from build123d import *

# Parameters (mm, degrees)
SKETCH1_W          = 300
SKETCH1_H          = 150
BLOCK_DEPTH        = 19.05
SKETCH3_W          = 250
SKETCH3_H          = 25
CUT_EXTRUDE2_DEPTH = 39.961179
SKETCH6_W          = 125
SKETCH6_H          = 20
CUT_EXTRUDE5_DEPTH = 20.05
SKETCH7_W          = 80
SKETCH7_H          = 50
CUT_EXTRUDE6_DEPTH = 20.05
SKETCH8_R          = 2
CUT_EXTRUDE7_DEPTH = 20.05


with BuildPart() as part:
    # Sketch1 → block (new body)
    with BuildSketch(Plane.XY):
        with Locations((150, 75)):
            Rectangle(SKETCH1_W, SKETCH1_H)
    extrude(amount=-BLOCK_DEPTH)

    # Sketch3 → Cut-Extrude2 (cut)
    with BuildSketch(Plane.XY):
        with Locations((150, 117.5)):
            Rectangle(SKETCH3_W, SKETCH3_H)
    extrude(amount=-CUT_EXTRUDE2_DEPTH, mode=Mode.SUBTRACT)

    # Sketch6 → Cut-Extrude5 (cut, through all)
    with BuildSketch(Plane.XY):
        with Locations((212.5, 95)):
            Rectangle(SKETCH6_W, SKETCH6_H)
    extrude(amount=-CUT_EXTRUDE5_DEPTH, mode=Mode.SUBTRACT)

    # Sketch7 → Cut-Extrude6 (cut, through all)
    with BuildSketch(Plane.XY):
        with Locations((200, 25)):
            Rectangle(SKETCH7_W, SKETCH7_H)
    extrude(amount=-CUT_EXTRUDE6_DEPTH, mode=Mode.SUBTRACT)

    # Sketch8 → Cut-Extrude7 (cut, through all)
    with BuildSketch(Plane.XY):
        with Locations((37.5875, 139.35)):
            Circle(SKETCH8_R)
        with Locations((82.0375, 139.35)):
            Circle(SKETCH8_R)
        with Locations((37.5875, 91.95)):
            Circle(SKETCH8_R)
        with Locations((82.0375, 91.95)):
            Circle(SKETCH8_R)
    extrude(amount=-CUT_EXTRUDE7_DEPTH, mode=Mode.SUBTRACT)


solid = part.part
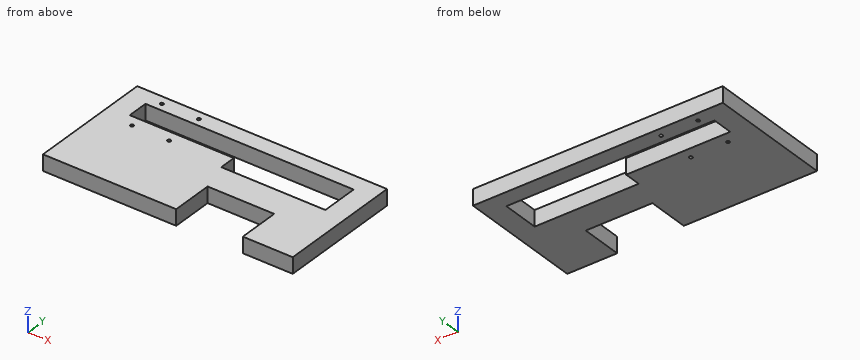
CAD build for the part. Positions are in the model's coordinates, mm. Coordinates: 2 decimals unless noted, no trailing zeros. Write each loop counter-clockwise with the first axis right and the second up, starting at its lowest first coordinate (ties: lowest second). Pieces come first, ordered by that corner, then holes. Notation, with made-up numbers: M 38.25,89.5 L 47.25,89.5 A20 ccw 47.25,102.5 Z; hole C 25.25,87 d9. An arc over 180 degrees is marked long. Answer as a JSON object with one key per item and string values. Group by question number.
1) Saw through at A-A (y = 23). Write the cut outline in (x, z), plus the area to 3 significant figures.
2) Saw through at B-B (x = 130.5). Write the cut outline in (y, z), plus the area to 3 significant figures.
3) Saw through at C-C (z = -9.5). Write the cut outline in (x, y).
4) Wall check: line 1 (X direction, y = 139.35, z = -12.25); line 2 (Y direction, x = 65.5, z = -9.75); line 3 (X direction, y = 99, z = -9). Give the ranges that are in metal, low to high. Write a range as from..to.
5) Pin check, flat tips, straight feed: pin 1 Ø5 at (x, y) = (37.59, 91.95) entering from -Z; pin 2 Ø8 at (x, y) = (248, 125.5) entering from +Z; pin 3 Ø5.5 at (x, z) = (215, -10.5) entering from -Y. Stop position of each tip, or through.
Values follow:
{
 "1": {"outline": "M 0,-19.05 L 160,-19.05 L 160,0 L 0,0 Z; M 240,-19.05 L 300,-19.05 L 300,0 L 240,0 Z", "area": "4,190 mm2"},
 "2": {"outline": "M 0,-19.05 L 105,-19.05 L 105,0 L 0,0 Z; M 130,-19.05 L 150,-19.05 L 150,0 L 130,0 Z", "area": "2,380 mm2"},
 "3": {"outline": "M 0,0 L 160,0 L 160,50 L 240,50 L 240,0 L 300,0 L 300,150 L 0,150 Z; hole M 25,105 L 150,105 L 150,85 L 275,85 L 275,130 L 25,130 Z; hole C 37.59,91.95 d4; hole C 37.59,139.35 d4; hole C 82.04,91.95 d4; hole C 82.04,139.35 d4"},
 "4": {"line 1": "x = 0..35.59, 39.59..80.04, 84.04..300", "line 2": "y = 0..105, 130..150", "line 3": "x = 0..150, 275..300"},
 "5": {"pin 1": "stops at z = -19.05", "pin 2": "passes through", "pin 3": "stops at y = 50"}
}
